```python
from build123d import *

# Parameters (mm, degrees)
BOSS_EXTRUDE1_DEPTH = 38.1
SKETCH4_R           = 6.35
CUT_EXTRUDE1_DEPTH  = 77.2
FILLET1_R           = 12.7
FILLET2_R           = 2.54


with BuildPart() as part:
    # Sketch1 → Boss-Extrude1 (new body)
    with BuildSketch(Plane(origin=(0, 0, 0), x_dir=(1, 0, 0), z_dir=(0, 1, 0))):
        Polygon((-5.55625, 27.9796875), (-5.55625, -10.1203125), (70.64375, -10.1203125), (70.64375, 27.9796875), (67.46875, 27.9796875), (67.46875, -6.9453125), (-2.38125, -6.9453125), (-2.38125, 27.9796875), align=None)
    extrude(amount=BOSS_EXTRUDE1_DEPTH)

    # Sketch4 → Cut-Extrude1 (cut, through all)
    with BuildSketch(Plane(origin=(70.64375, 0, 0), x_dir=(0, 0, -1), z_dir=(1, 0, 0))):
        with Locations((8.9296875, 19.05)):
            Circle(SKETCH4_R)
    extrude(amount=-CUT_EXTRUDE1_DEPTH, mode=Mode.SUBTRACT)

    # Fillet1
    fillet1_edges = [part.edges().sort_by_distance(p)[0] for p in [
        (-3.96875, 0, -27.9796875),
        (69.05625, 38.1, -27.9796875),
        (-3.96875, 38.1, -27.9796875),
        (69.05625, 0, -27.9796875),
    ]]
    fillet(fillet1_edges, radius=FILLET1_R)

    # Fillet2
    fillet2_edges = [part.edges().sort_by_distance(p)[0] for p in [
        (-2.38125, 19.05, 6.9453125),
        (67.46875, 19.05, 6.9453125),
        (70.64375, 19.05, 10.1203125),
        (-5.55625, 19.05, 10.1203125),
    ]]
    fillet(fillet2_edges, radius=FILLET2_R)


solid = part.part
```
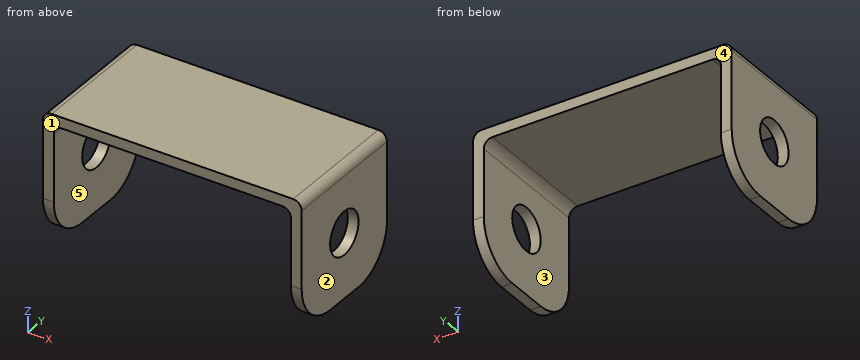
The listing builds one solid part. Answer for the finished solid, in the listing's coordinates (mm). Face numbers are marked on the shaded views. A direction names the side the tool comes from. Give positions to 0.01 mm unless a question says otherwise; leave off trailing zeros. Order: outer loops, then holes, each group sorted by start corner. A loop starts at its lowest first (then second) coordinate and runs counter-clockwise, first axis right, second up. Notation, with made-up numbers: (-6, 26) -> (6, 26) arc R25 cw to (6, 54) -> close; hole circle Ø7 at (-13.75, 84.25). An arc over 180 degrees is marked (long way). Answer as a JSON object with one key per item and string values. Group by question number.
Item 1: A tool of negligible diameter and unlimited length cuts with its end or side. For the marked faces 4 and 5, from which of +Z, -Z, +X, -X, +Y, -Y can it reach the whole face along a straight path? Write none if from no direction.
Item 2: Determine the mould class of the marked faces 1, 2 and 3 for opening direction X: pulls with the +X half, pulls with the -X half, needs draft (parallel to the pull), parting line crosses it, or undercut.
Item 3: The part is cut by section B-B on y = 19.05. Write down the section's boundary in (x, z).
Item 4: The part is cut by section A-A on z = 1. Write down the section's boundary in (x, y), and give its area (3 significant figures).
Item 5: The part is cut by section C-C on z = -4.5. Write down the section's boundary in (x, y), and give its area (3 significant figures).
Item 6: A flat-ended cylindrical pin translates along its axis: pin 1 (3 mm diameter, centred on x = 57, y = 22.5, fed in from -Z). Find the tip coordinate at first contact, or state that the pin passes through.
Item 7: The part is cut by section D-D on y = 10. Write down the section's boundary in (x, z).
Item 8: Consider L1, parallel to Z at x = 68, y = 19; L2, parallel to X at y = 6, z = 1; L3, parallel to Z at x = 31.5, y = 4.5. Determine where each line is inside the solid, lowest interval first. Write a range as from..to.
Result set:
{
 "1": {"face 4": "+Z, -Z, +X, -X, +Y", "face 5": "-Z, +Y, -Y"},
 "2": {"face 1": "needs draft", "face 2": "pulls with the +X half", "face 3": "undercut"},
 "3": {"outline": "(-5.56, -27.98) -> (-2.38, -27.98) -> (-2.38, -15.28) -> (-5.56, -15.28) -> close; (-5.56, -2.58) -> (-2.38, -2.58) -> (-2.38, 4.41) arc R2.54 cw to (0.16, 6.95) -> (64.93, 6.95) arc R2.54 cw to (67.47, 4.41) -> (67.47, -2.58) -> (70.64, -2.58) -> (70.64, 7.58) arc R2.54 ccw to (68.1, 10.12) -> (-3.02, 10.12) arc R2.54 ccw to (-5.56, 7.58) -> close; (67.47, -27.98) -> (70.64, -27.98) -> (70.64, -15.28) -> (67.47, -15.28) -> close"},
 "4": {"outline": "(-5.56, 0) -> (-2.38, 0) -> (-2.38, 38.1) -> (-5.56, 38.1) -> close; (67.47, 0) -> (70.64, 0) -> (70.64, 38.1) -> (67.47, 38.1) -> close", "area": "242 mm²"},
 "5": {"outline": "(-5.56, 0) -> (-2.38, 0) -> (-2.38, 14.5) -> (-5.56, 14.5) -> close; (-5.56, 23.6) -> (-2.38, 23.6) -> (-2.38, 38.1) -> (-5.56, 38.1) -> close; (67.47, 0) -> (70.64, 0) -> (70.64, 14.5) -> (67.47, 14.5) -> close; (67.47, 23.6) -> (70.64, 23.6) -> (70.64, 38.1) -> (67.47, 38.1) -> close", "area": "184 mm²"},
 "6": {"pin 1": "z = 6.95"},
 "7": {"outline": "(-5.56, -27.69) -> (-2.38, -27.69) -> (-2.38, 4.41) arc R2.54 cw to (0.16, 6.95) -> (64.93, 6.95) arc R2.54 cw to (67.47, 4.41) -> (67.47, -27.69) -> (70.64, -27.69) -> (70.64, 7.58) arc R2.54 ccw to (68.1, 10.12) -> (-3.02, 10.12) arc R2.54 ccw to (-5.56, 7.58) -> close"},
 "8": {"L1": "-27.98..-15.28, -2.58..10.12", "L2": "-5.56..-2.38, 67.47..70.64", "L3": "6.95..10.12"}
}
